from build123d import *

# Parameters (mm, degrees)
SKETCH1_R                 = 33
BOSS_EXTRUDE1_DEPTH       = 4
SKETCH2_R                 = 33
SKETCH2_R_2               = 31
BOSS_EXTRUDE2_DEPTH       = 16.88
M2_CLEARANCE_HOLE1_D      = 2.4
SKETCH13_R                = 2.5
CUT_EXTRUDE3_DEPTH        = 5
CUT_EXTRUDE2_DEPTH        = 5
SKETCH15_R                = 3
BOSS_EXTRUDE3_DEPTH       = 20.88
FILLET1_R                 = 5
CIRPATTERN1_COUNT         = 4
FILLET1_OF_CIRPATTERN1_R  = 5
M3X0_5_TAPPED_HOLE1_D     = 2.5
M3X0_5_TAPPED_HOLE1_DEPTH = 7.5
M3X0_5_TAPPED_HOLE1_TIP   = 0.751075774


with BuildPart() as part:
    # Sketch1 → Boss-Extrude1 (new body)
    with BuildSketch(Plane(origin=(0, 0, 0), x_dir=(1, 0, 0), z_dir=(0, 1, 0))):
        Circle(SKETCH1_R)
    extrude(amount=BOSS_EXTRUDE1_DEPTH)

    # Sketch2 → Boss-Extrude2 (add)
    with BuildSketch(Plane(origin=(0, 4, 0), x_dir=(1, 0, 0), z_dir=(0, 1, 0))):
        Circle(SKETCH2_R)
        Circle(SKETCH2_R_2, mode=Mode.SUBTRACT)
    extrude(amount=BOSS_EXTRUDE2_DEPTH)

    # M2 Clearance Hole1 (through all)
    with Locations(Plane(origin=(0, 0, 0), x_dir=(-1, 0, 0), z_dir=(0, -1, 0))):
        with Locations((3.181980515, 3.181980515), (3.181980515, -3.181980515), (-3.181980515, -3.181980515), (-3.181980515, 3.181980515)):
            Hole(M2_CLEARANCE_HOLE1_D / 2)

    # Sketch13 → Cut-Extrude3 (cut, through all)
    with BuildSketch(Plane(origin=(0, 4, 0), x_dir=(1, 0, 0), z_dir=(0, 1, 0))):
        Circle(SKETCH13_R)
    extrude(amount=-CUT_EXTRUDE3_DEPTH, mode=Mode.SUBTRACT)

    # Sketch10 → Cut-Extrude2 (cut, through all)
    with BuildSketch(Plane(origin=(0, 4, 0), x_dir=(1, 0, 0), z_dir=(0, 1, 0))):
        with BuildLine():
            Line((13.5, -4), (13.5, 4))
            ThreePointArc((13.5, 4), (15, 5.5), (16.5, 4))
            Line((16.5, 4), (16.5, -4))
            ThreePointArc((16.5, -4), (15, -5.5), (13.5, -4))
        make_face()
    extrude(amount=-CUT_EXTRUDE2_DEPTH, mode=Mode.SUBTRACT)

    # Sketch15 → Boss-Extrude3 (add, through all)
    with BuildSketch(Plane(origin=(0, 20.88, 0), x_dir=(1, 0, 0), z_dir=(0, 1, 0))):
        with Locations((24.04163056, 24.04163056)):
            Circle(SKETCH15_R)
    boss_extrude3 = extrude(amount=-BOSS_EXTRUDE3_DEPTH)

    # Fillet1
    fillet1_edges = [part.edges().sort_by_distance(p)[0] for p in [
        (25.219946573, 10.44, -21.282722919),
        (21.282722919, 10.44, -25.219946573),
    ]]
    fillet(fillet1_edges, radius=FILLET1_R)

    # CirPattern1: Boss-Extrude3 ×4 about axis
    cirpattern1_axis = Axis((0, 0, 0), (0, 1, 0))
    for i in range(1, CIRPATTERN1_COUNT):
        add(boss_extrude3.rotate(cirpattern1_axis, i * 360 / CIRPATTERN1_COUNT))

    # Fillet1 of CirPattern1
    fillet1_of_cirpattern1_edges = [part.edges().sort_by_distance(p)[0] for p in [
        (-21.282722919, 10.44, -25.219946573),
        (-25.219946573, 10.44, -21.282722919),
        (-25.219946573, 10.44, 21.282722919),
        (-21.282722919, 10.44, 25.219946573),
        (21.282722919, 10.44, 25.219946573),
        (25.219946573, 10.44, 21.282722919),
    ]]
    fillet(fillet1_of_cirpattern1_edges, radius=FILLET1_OF_CIRPATTERN1_R)

    # M3x0.5 Tapped Hole1
    with Locations(Plane(origin=(0, 20.88, 0), x_dir=(1, 0, 0), z_dir=(0, 1, 0))):
        with Locations((24.04163056, -24.04163056), (-24.04163056, -24.04163056), (-24.04163056, 24.04163056), (24.04163056, 24.04163056)):
            Hole(M3X0_5_TAPPED_HOLE1_D / 2, depth=M3X0_5_TAPPED_HOLE1_DEPTH)
            with Locations((0, 0, -(M3X0_5_TAPPED_HOLE1_DEPTH + M3X0_5_TAPPED_HOLE1_TIP / 2))):  # 118° drill point
                Cone(0, M3X0_5_TAPPED_HOLE1_D / 2, M3X0_5_TAPPED_HOLE1_TIP, mode=Mode.SUBTRACT)


solid = part.part
Model file for the job. Use its own axes, mm. A direction names the side the tool comes from. Round coordinates to 2 decimals unless told otherwise and drop trailing zeros. Loops run counter-clockwise (first coordinate to the right, second up) from the corner with the lowest first, then second, coordinate; pieces in that order, holes last. Notation, with made-up numbers: (57, -27.75) - (115, -27.75) arc R22 ccw to (115, -11.75) - close; hole circle Ø3 at (23, 64). An arc over 180 degrees is marked (long way). Write each question's results on one line, items separated by ' | '.
(1) Pin check, flat tips, straight feed: pin 1 (10 mm diameter, centred on y = 5.5, z = 17.5, fed in from -X); pin 2 (4 mm diameter, centred on y = 11, z = 3.5, fed in from -X); pin 3 (8 mm diameter, centred on x = -4, z = -17.5, fed in from +Y). Stop position of each tip, or through.
Answer below:
pin 1: stops at x = -30.54 | pin 2: stops at x = -32.97 | pin 3: stops at y = 4
(2) 3-axis set-ups, long thin cutter, end or side, ignore diameter. For faces 1 (the cylindrical face through (-4.036, 12.322, -30.736)), 2 (the cylindrical face through (0, 10, 33)), 3 (the cylindrical face through (15, 2, 5.5)): which of +Z, -Z, +X, -X, +Y, -Y reach the whole face in a straight line?
Answer below:
face 1: +Y | face 2: +Z, +Y, -Y | face 3: +Y, -Y
(3) Saw through at C-C, the plane y = 17.25. Count the separate pieces of the cut face and the enclosed holes in it, then the cut area to 3 significant figures.
Answer below:
separate pieces: 1 | enclosed holes: 5 | area: 479 mm^2
(4) Saw through at B-B, the plane x = -9. List the corners of the cut face in (y, z), then the cut area to 3 significant figures.
Answer below:
outline: (0, -31.75) - (20.88, -31.75) - (20.88, -29.66) - (4, -29.66) - (4, 29.66) - (20.88, 29.66) - (20.88, 31.75) - (0, 31.75) - close | area: 324 mm^2
(5) Saw through at D-D, the plane z = -9. List the corners of the cut face in (x, y), then the cut area to 3 significant figures.
Answer below:
outline: (-31.75, 0) - (31.75, 0) - (31.75, 20.88) - (29.66, 20.88) - (29.66, 4) - (-29.66, 4) - (-29.66, 20.88) - (-31.75, 20.88) - close | area: 324 mm^2
(6) Saw through at A-A, the plane x = 0. List the corners of the cut face in (y, z).
Answer below:
outline: (0, -33) - (20.88, -33) - (20.88, -31) - (4, -31) - (4, -2.5) - (0, -2.5) - close; (0, 2.5) - (4, 2.5) - (4, 31) - (20.88, 31) - (20.88, 33) - (0, 33) - close
(7) Mould opens along X. For faces 4 (the cylindrical face through (0, 10, -33)), 5 (the cylindrical face through (33, 10, 0)), 6 (the conical face through (-24.214, 12.759, -23.91)) say: released by +X, released by -X, zero draft, split by the parting line, or undercut.
Answer below:
face 4: split by the parting line | face 5: released by +X | face 6: undercut
(8) Wall check: L1, parallel to X at y = 1.85, z = 0; L2, parallel to X at y = 4.5, z = 0.5; L3, parallel to Y at x = 23.5, z = -7. Give the ranges that are in metal, low to high.
Answer below:
L1: x = -33 to -2.5, 2.5 to 13.5, 16.5 to 33 | L2: x = -33 to -31, 31 to 33 | L3: y = 0 to 4
